```python
from build123d import *

# Parameters (mm, degrees)
SKETCH1_W                                           = 45
SKETCH1_H                                           = 20
BOSS_EXTRUDE1_DEPTH                                 = 25
SKETCH2_W                                           = 12
SKETCH2_H                                           = 25
BOSS_EXTRUDE2_DEPTH                                 = 40
SKETCH3_R                                           = 1.75
CUT_EXTRUDE1_DEPTH                                  = 61.259853966
SKETCH4_R                                           = 1.75
CUT_EXTRUDE2_DEPTH                                  = 25
CBORE_FOR_M3_HEX_SOCKET_HEAD_CAP_SCREW1_D           = 3.5
CBORE_FOR_M3_HEX_SOCKET_HEAD_CAP_SCREW1_CBORE_D     = 6.5
CBORE_FOR_M3_HEX_SOCKET_HEAD_CAP_SCREW1_CBORE_DEPTH = 11.4
CBORE_FOR_M3_HEX_SOCKET_HEAD_CAP_SCREW2_D           = 3.5
CBORE_FOR_M3_HEX_SOCKET_HEAD_CAP_SCREW2_CBORE_D     = 6.5
CBORE_FOR_M3_HEX_SOCKET_HEAD_CAP_SCREW2_CBORE_DEPTH = 4
CBORE_FOR_M3_PAN_HEAD_SCREW1_D                      = 3.5
CBORE_FOR_M3_PAN_HEAD_SCREW1_CBORE_D                = 6.5
CBORE_FOR_M3_PAN_HEAD_SCREW1_CBORE_DEPTH            = 12.4
CUT_EXTRUDE3_DEPTH                                  = 72.763500472
CUT_EXTRUDE3_DEPTH_BACK                             = 72.763500472
SKETCH9_W                                           = 12
SKETCH9_H                                           = 14
SKETCH10_W                                          = 12
SKETCH10_H                                          = 8
SKETCH10_H_2                                        = 3
CUT_EXTRUDE5_DEPTH                                  = 1
FILLET2_R                                           = 5
FILLET5_R                                           = 3
SKETCH13_R                                          = 11.25
CUT_EXTRUDE6_DEPTH                                  = 2.5


with BuildPart() as part:
    # Sketch1 → Boss-Extrude1 (new body)
    with BuildSketch(Plane(origin=(0, 0, 0), x_dir=(1, 0, 0), z_dir=(0, 1, 0))):
        Rectangle(SKETCH1_W, SKETCH1_H)
    extrude(amount=BOSS_EXTRUDE1_DEPTH)

    # Sketch2 → Boss-Extrude2 (add)
    with BuildSketch(Plane(origin=(0, 0, -10), x_dir=(-1, 0, 0), z_dir=(0, 0, -1))):
        with Locations((-16.5, 12.5)):
            Rectangle(SKETCH2_W, SKETCH2_H)
        with Locations((16.5, 12.5)):
            Rectangle(SKETCH2_W, SKETCH2_H)
    extrude(amount=BOSS_EXTRUDE2_DEPTH)

    # Sketch3 → Cut-Extrude1 (cut, through all)
    with BuildSketch(Plane(origin=(0, 25, 0), x_dir=(1, 0, 0), z_dir=(0, 1, 0))):
        with Locations(Location((15.5, 44, 0), (0, 0, 270))):
            Circle(SKETCH3_R)
        with Locations(Location((15.5, 13, 0), (0, 0, 270))):
            Circle(SKETCH3_R)
        with Locations(Location((-15.5, 13, 0), (0, 0, 270))):
            Circle(SKETCH3_R)
        with Locations(Location((-15.5, 44, 0), (0, 0, 270))):
            Circle(SKETCH3_R)
    extrude(amount=-CUT_EXTRUDE1_DEPTH, mode=Mode.SUBTRACT)

    # Sketch4 → Cut-Extrude2 (cut)
    with BuildSketch(Plane(origin=(0, 25, 0), x_dir=(1, 0, 0), z_dir=(0, 1, 0))):
        with Locations(Location((-15.5, 0, 0), (0, 0, 270))):
            Circle(SKETCH4_R)
        with Locations(Location((15.5, 0, 0), (0, 0, 270))):
            Circle(SKETCH4_R)
    extrude(amount=-CUT_EXTRUDE2_DEPTH, mode=Mode.SUBTRACT)

    # CBORE for M3 Hex Socket Head Cap Screw1 (through all)
    with Locations(Plane(origin=(0, 25, 0), x_dir=(1, 0, 0), z_dir=(0, 1, 0))):
        with Locations((15.5, 0), (-15.5, 0)):
            CounterBoreHole(CBORE_FOR_M3_HEX_SOCKET_HEAD_CAP_SCREW1_D / 2, CBORE_FOR_M3_HEX_SOCKET_HEAD_CAP_SCREW1_CBORE_D / 2, CBORE_FOR_M3_HEX_SOCKET_HEAD_CAP_SCREW1_CBORE_DEPTH)

    # CBORE for M3 Hex Socket Head Cap Screw2 (through all)
    with Locations(Plane(origin=(0, 0, 0), x_dir=(-1, 0, 0), z_dir=(0, -1, 0))):
        with Locations((15.5, 44), (15.5, 13), (-15.5, 13), (-15.5, 44)):
            CounterBoreHole(CBORE_FOR_M3_HEX_SOCKET_HEAD_CAP_SCREW2_D / 2, CBORE_FOR_M3_HEX_SOCKET_HEAD_CAP_SCREW2_CBORE_D / 2, CBORE_FOR_M3_HEX_SOCKET_HEAD_CAP_SCREW2_CBORE_DEPTH)

    # CBORE for M3 Pan Head Screw1 (through all)
    with Locations(Plane(origin=(0, 0, 0), x_dir=(-1, 0, 0), z_dir=(0, -1, 0))):
        with Locations((-15.5, 13), (15.5, 13)):
            CounterBoreHole(CBORE_FOR_M3_PAN_HEAD_SCREW1_D / 2, CBORE_FOR_M3_PAN_HEAD_SCREW1_CBORE_D / 2, CBORE_FOR_M3_PAN_HEAD_SCREW1_CBORE_DEPTH)

    # Sketch9 → Cut-Extrude3 (cut, two sides: drawn at the far end of the back side and taken through both)
    with BuildSketch(Plane(origin=(22.5, 0, 0), x_dir=(0, 0, -1), z_dir=(1, 0, 0)).offset(-CUT_EXTRUDE3_DEPTH_BACK)):
        with Locations((44, 15)):
            Rectangle(SKETCH9_W, SKETCH9_H)
    extrude(amount=CUT_EXTRUDE3_DEPTH + CUT_EXTRUDE3_DEPTH_BACK, mode=Mode.SUBTRACT)

    # Sketch10 → Cut-Extrude5 (cut)
    with BuildSketch(Plane(origin=(0, 0, -50), x_dir=(-1, 0, 0), z_dir=(0, 0, -1))):
        with Locations((-16.5, 4)):
            Rectangle(SKETCH10_W, SKETCH10_H)
        with Locations((16.5, 4)):
            Rectangle(SKETCH10_W, SKETCH10_H)
        with Locations((-16.5, 23.5)):
            Rectangle(SKETCH10_W, SKETCH10_H_2)
        with Locations((16.5, 23.5)):
            Rectangle(SKETCH10_W, SKETCH10_H_2)
    extrude(amount=-CUT_EXTRUDE5_DEPTH, mode=Mode.SUBTRACT)

    # Fillet2
    fillet2_edges = [part.edges().sort_by_distance(p)[0] for p in [
        (-10.5, 4, -49),
        (-22.5, 4, -49),
        (22.5, 23.5, -49),
        (10.5, 23.5, -49),
        (-10.5, 23.5, -49),
        (-22.5, 23.5, -49),
        (22.5, 4, -49),
        (10.5, 4, -49),
    ]]
    fillet(fillet2_edges, radius=FILLET2_R)

    # Fillet5
    fillet5_edges = [part.edges().sort_by_distance(p)[0] for p in [
        (-10.5, 15, -38),
        (10.5, 15, -38),
    ]]
    fillet(fillet5_edges, radius=FILLET5_R)

    # Sketch13 → Cut-Extrude6 (cut)
    with BuildSketch(Plane(origin=(0, 25, 0), x_dir=(1, 0, 0), z_dir=(0, 1, 0))):
        with Locations((0, 28.5)):
            Circle(SKETCH13_R)
    extrude(amount=-CUT_EXTRUDE6_DEPTH, mode=Mode.SUBTRACT)


solid = part.part
```
Check sheet for the modelled part. Datum: model origin and axes. Units: mm. A direction names the side the tool comes from. Give positions to 0.01 mm unless a question says otherwise; leave off trailing zeros. Write each loop counter-clockwise with the first axis right and the second up, starting at its lowest first coordinate (ties: lowest second). Pieces come first, ordered by that corner, then holes.
Item 1: Draft check along Z on faces 4 (the face through (-17, 8, -42)), 5 (the face through (-14, 6.9, 0.9)), 6 (the face through (-14.795, 1.972, -40.827)), 7 (the face through (11.4, 14.9, -37.14)). Enter one of: released by +Z, released by -Z, zero draft, split by the parting line, or undercut.
Item 2: Cross-section at B-B (y = 2.5). Enter the section's corners in (x, z), and give its area (3 significant figures).
Item 3: Cross-section at A-A (z = -13). Enter the section's corners in (x, y).
Item 4: Scan lines: L1, parallel to X at y = 8.25, z = 0; L2, parallel to Z at x = 15.5, y = 23.3; L3, parallel to Z at x = -15.5, y = 3.5. Record each from-to range of solid material in increasing order.
Item 5: Gauge pin test, flat ends, axial feed: pin 1 (3 mm diameter, centred on x = 15, z = -11.5, fed in from -Y); pin 2 (4.5 mm diameter, centred on x = -17, y = 13.5, fed in from -Z); pin 3 (6 mm diameter, centred on x = 15, z = -41.5, fed in from -Y); pin 4 (4.5 mm diameter, centred on x = -15.5, z = -44, fed in from -Y). Record the tip position at first contact, or that the pin passes through.
Item 6: Cross-section at C-C (y = 10). Enter the section's corners in (x, z), and give its area (3 significant figures).
Item 7: Access from +Z, -Z, +X, -X, +Y, -Y to the whole of each face (thin tool, end or side, straight path). Record for faces 1 (the face through (-14.1, 13.6, 1.4)), 2 (the face through (12, 4.06, -47.57)), 3 (the face through (-16.9, 12.4, -11.6)).
Item 8: Cross-section at D-D (z = -29.5). Enter the section's corners in (x, y), and give its area (3 significant figures).
Report:
1. face 4: zero draft
1. face 5: undercut
1. face 6: undercut
1. face 7: released by -Z
2. outline: (-22.5, -44) arc R5 ccw to (-17.5, -49) - (-15.5, -49) arc R5 ccw to (-10.5, -44) - (-10.5, -10) - (10.5, -10) - (10.5, -44) arc R5 ccw to (15.5, -49) - (17.5, -49) arc R5 ccw to (22.5, -44) - (22.5, 10) - (-22.5, 10) - close; hole circle Ø6.5 at (-15.5, -44); hole circle Ø6.5 at (-15.5, -13); hole circle Ø3.5 at (-15.5, 0); hole circle Ø6.5 at (15.5, -44); hole circle Ø6.5 at (15.5, -13); hole circle Ø3.5 at (15.5, 0)
2. area: 1,660 mm2
3. outline: (-22.5, 0) - (-18.75, 0) - (-18.75, 12.4) - (-17.25, 12.4) - (-17.25, 25) - (-22.5, 25) - close; (-13.75, 12.4) - (-12.25, 12.4) - (-12.25, 0) - (-10.5, 0) - (-10.5, 25) - (-13.75, 25) - close; (10.5, 0) - (12.25, 0) - (12.25, 12.4) - (13.75, 12.4) - (13.75, 25) - (10.5, 25) - close; (17.25, 12.4) - (18.75, 12.4) - (18.75, 0) - (22.5, 0) - (22.5, 25) - (17.25, 25) - close
4. L1: x = -22.5 to -17.25, -13.75 to 13.75, 17.25 to 22.5
4. L2: z = -49 to -45.75, -42.25 to -14.75, -11.25 to -3.25, 3.25 to 10
4. L3: z = -49 to -47.25, -40.75 to -16.25, -9.75 to -1.75, 1.75 to 10
5. pin 1: stops at y = 12.4
5. pin 2: stops at z = -38
5. pin 3: stops at y = 0
5. pin 4: stops at y = 4
6. outline: (-22.5, -38) - (-13.5, -38) arc R3 ccw to (-10.5, -35) - (-10.5, -10) - (10.5, -10) - (10.5, -35) arc R3 ccw to (13.5, -38) - (22.5, -38) - (22.5, 10) - (-22.5, 10) - close; hole circle Ø6.5 at (-15.5, -13); hole circle Ø3.5 at (-15.5, 0); hole circle Ø6.5 at (15.5, -13); hole circle Ø3.5 at (15.5, 0)
6. area: 1,480 mm2
7. face 1: +Y
7. face 2: -Z, +Y, -Y
7. face 3: -Y
8. outline: (-22.5, 0) - (-10.5, 0) - (-10.5, 22.5) - (-11.21, 22.5) - (-11.21, 25) - (-22.5, 25) - close; (10.5, 0) - (22.5, 0) - (22.5, 25) - (11.21, 25) - (11.21, 22.5) - (10.5, 22.5) - close
8. area: 596 mm2
